from build123d import *

# Parameters (mm, degrees)
F0_R          = 28.575
F1_DEPTH      = 76.2
F1_DEPTH_BACK = 76.2
F2_R          = 22.225
F2_R_2        = 19.05
F3_DEPTH      = 76.2
F4_R          = 25.4
F5_DEPTH      = 152.4


with BuildPart() as f1:
    # F0 (on Right) → F1 (new body, two sides)
    with BuildSketch(Plane.YZ) as f1_sk:
        Circle(F0_R)
    extrude(amount=F1_DEPTH)
    extrude(f1_sk.sketch, amount=-F1_DEPTH_BACK)

    # F2 (on Front) → F3 (join)
    with BuildSketch(Plane.XZ):
        Circle(F2_R)
        Circle(F2_R_2, mode=Mode.SUBTRACT)
    extrude(amount=F3_DEPTH)

    # F4 (on face) → F5 (cut)
    with BuildSketch(Plane.YZ.offset(76.2)):
        Circle(F4_R)
    extrude(amount=-F5_DEPTH, mode=Mode.SUBTRACT)


solid = f1.part
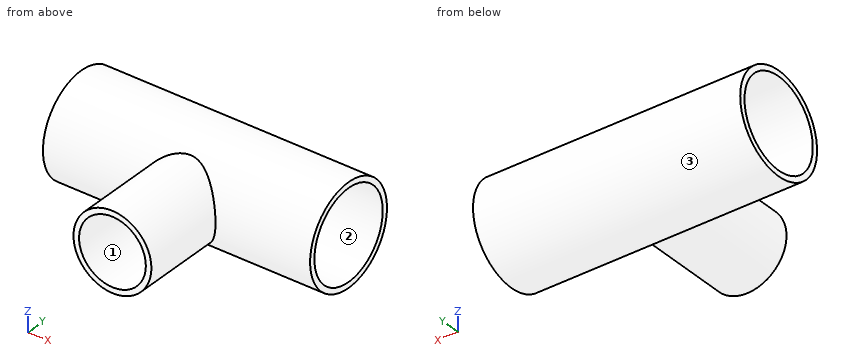
Can you work these out from the model? Positions are in its coordinate system, mm. Face numbers are marked on the shaded views. Give positions to 0.01 mm unless a question says otherwise; leave off trailing zeros. Write each loop counter-clockwise with the first axis right and the second up, starting at its lowest first coordinate (ties: lowest second). Pieces come first, ordered by that corner, then holes. Notation, with made-up numbers: M -32,70.5 L -15,70.5 A10 cw -15,88.5 Z; hole C 42,19 d1. An arc over 180 degrees is marked long. Answer in a Markdown table with one row per item. Add a question column.
Item 1: Imagine slicing it at B-B, the plane x = 0. Write out the boundary of the cut face in (y, z) (3 decimals).
Item 2: Imagine slicing it at C-C, the plane y = 0. Write out the boundary of the cut face in (x, z) (3 decimals), plus the area to 3 significant figures.
Item 3: For pin 1 Ø3 at (x, z) = (-39, -11.5) entering from -Y; pin 2 Ø1 at (x, z) = (-18, -20) entering from +Y; pin 3 Ø4 at (y, z) = (-57.5, -20) entering from +X, each with a flat end and sliding along its axis, tell me the tip position at first contact or that it passes through.
Item 4: We'd pull the mould along Y, two halves only. Please class the marked faces 1, 2 and 3: released by +Y, released by -Y, zero draft, split by the parting line, or undercut.
Item 5: Imagine slicing it at D-D, the plane y = -38. Write out the boundary of the cut face in (x, z) (3 decimals).
Item 6: Imagine slicing it at A-A, the plane z = 0. Write out the boundary of the cut face in (x, y) (3 decimals).
Item 7: Please list where these lines run through material, in increasing order: L1, parallel to Z at x = -31, y = 0 (3 decimals); L2, parallel to Z at x = 0, y = -35.5 (3 decimals); L3, parallel to X at y = -67.5, z = 1.
Evaluation:
| question | item | result |
|---|---|---|
| 1 | outline | M -76.2,-22.225 L -17.961,-22.225 A28.575 ccw long -17.961,22.225 L -76.2,22.225 L -76.2,19.05 L -21.299,19.05 A28.575 ccw -21.299,-19.05 L -76.2,-19.05 Z; hole C 0,0 d50.8 |
| 2 | outline | M -76.2,-28.575 L 76.2,-28.575 L 76.2,-25.4 L -76.2,-25.4 Z; M -76.2,25.4 L 76.2,25.4 L 76.2,28.575 L -76.2,28.575 Z |
| 2 | area | 968 mm² |
| 3 | pin 1 | stops at y = -26.77 |
| 3 | pin 2 | stops at y = 20.89 |
| 3 | pin 3 | stops at x = 13.04 |
| 4 | face 1 | zero draft |
| 4 | face 2 | undercut |
| 4 | face 3 | split by the parting line |
| 5 | outline | C 0,0 d44.45; hole C 0,0 d38.1 |
| 6 | outline | M -76.2,-28.575 L -22.225,-28.575 L -22.225,-76.2 L -19.05,-76.2 L -19.05,-28.575 L 19.05,-28.575 L 19.05,-76.2 L 22.225,-76.2 L 22.225,-28.575 L 76.2,-28.575 L 76.2,-25.4 L -76.2,-25.4 Z; M -76.2,25.4 L 76.2,25.4 L 76.2,28.575 L -76.2,28.575 Z |
| 7 | L1 | z = -28.575 to -25.4, 25.4 to 28.575 |
| 7 | L2 | z = -22.225 to -19.05, 19.05 to 22.225 |
| 7 | L3 | x = -22.2 to -19.02, 19.02 to 22.2 |
